CAD build for the part. Positions are in the model's coordinates, mm. Coordinates: 2 decimals unless noted, no trailing zeros. Order: outer loops, then holes, each group sorted by start corner. A loop starts at its lowest first (then second) coordinate and runs counter-clockwise, first axis right, second up. Notation, with made-up numbers: (50.5, 87.25) - (106.5, 87.25) arc R9 cw to (106.5, 93.25) - close; hole circle Ø10 at (53.25, 40). An arc over 180 degrees is marked (long way). Use one line per item in the form item = value.
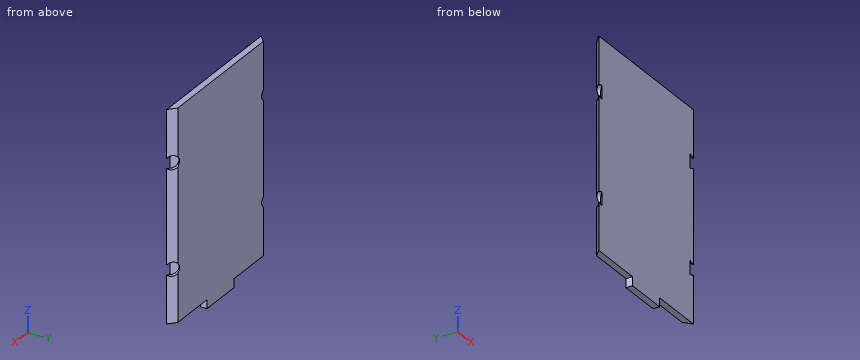
```python
from build123d import *

# Parameters (mm, degrees)
BOSS_EXTRUDE1_DEPTH = 120.65
SKETCH2_W           = 25.4
SKETCH2_H           = 5.08
BOSS_EXTRUDE2_DEPTH = 3.81
SKETCH3_R           = 4
CUT_EXTRUDE1_DEPTH  = 2
SKETCH4_R           = 4
CUT_EXTRUDE2_DEPTH  = 2


with BuildPart() as part:
    # Sketch1 → Boss-Extrude1 (new body)
    with BuildSketch(Plane.XY):
        Polygon((-40.203883769, 5.937788296), (40.203883769, 5.937788296), (44.399042974, 2.127788296), (-44.399042974, 2.127788296), align=None)
    extrude(amount=BOSS_EXTRUDE1_DEPTH)

    # Sketch2 → Boss-Extrude2 (add)
    with BuildSketch(Plane.XZ.offset(-2.127788296)):
        with Locations((0, -2.54)):
            Rectangle(SKETCH2_W, SKETCH2_H)
    extrude(amount=-BOSS_EXTRUDE2_DEPTH)

    # Sketch3 → Cut-Extrude1 (cut)
    with BuildSketch(Plane(origin=(-21.127225221, 23.263011377, 0), x_dir=(0.7402720771062569, 0.6723074087475075, 0), z_dir=(-0.6723074087475075, 0.7402720771062569, 0))):
        with Locations((-28.603318705, -30.353)):
            Circle(SKETCH3_R)
        with Locations((-28.603318705, -90.297)):
            Circle(SKETCH3_R)
    extrude(amount=-CUT_EXTRUDE1_DEPTH, mode=Mode.SUBTRACT)

    # Sketch4 → Cut-Extrude2 (cut)
    with BuildSketch(Plane(origin=(21.127225221, 23.263011377, 0), x_dir=(0.7402720771062569, -0.6723074087475075, 0), z_dir=(0.6723074087475075, 0.7402720771062569, 0))):
        with Locations((28.603318705, -90.297)):
            Circle(SKETCH4_R)
        with Locations((28.603318705, -30.353)):
            Circle(SKETCH4_R)
    extrude(amount=-CUT_EXTRUDE2_DEPTH, mode=Mode.SUBTRACT)


solid = part.part
```
Item 1: Drill centre lines: line 1 (Z direction, x = -28.5, y = 4.2); line 2 (X direction, y = 2.4, z = 14.5); line 3 (X direction, y = 5.55, z = 92). Where is each one in solid material? Low to high. Write a range as [from, to].
Derived:
line_1 = [0, 120.65]
line_2 = [-44.1, 44.1]
line_3 = [-38.79, 38.79]
Item 2: Cut at A-A, the plane x = 29. Write the cut outline in (y, z), plus the area to 3 significant figures.
Derived:
outline = (2.13, 0) - (5.94, 0) - (5.94, 120.65) - (2.13, 120.65) - close
area = 460 mm²
Item 3: Cut at B-B, the plane z = 51.5. Write the cut outline in (x, y).
Derived:
outline = (-44.4, 2.13) - (44.4, 2.13) - (40.2, 5.94) - (-40.2, 5.94) - close
Item 4: Drop flat-ended pins along their axis: pin 1 (1.9 mm diameter, centred on y = 4, z = -2, fed in from +X); pin 2 (1.1 mm diameter, centred on y = 5, z = -2, fed in from -X); pin 3 (1.1 mm diameter, centred on x = 30.5, y = 4, fed in from -Z). Give the stop position or say it passes through.
Derived:
pin_1 = 12.7
pin_2 = -12.7
pin_3 = 0
